from build123d import *

# Parameters (mm, degrees)
SKETCH1_R             = 41
BOSS_EXTRUDE1_DEPTH   = 34
SKETCH2_R             = 35
CUT_EXTRUDE1_DEPTH    = 21
CUT_EXTRUDE2_DEPTH    = 21
SKETCH6_R             = 11
BOSS_EXTRUDE2_DEPTH   = 26
ESBO_O1_R             = 3.25
CORTE_EXTRUS_O1_DEPTH = 15
ESBO_O2_W             = 0.9
ESBO_O2_H             = 31
CORTE_EXTRUS_O4_DEPTH = 12.8


with BuildPart() as part:
    # Sketch1 → Boss-Extrude1 (new body)
    with BuildSketch(Plane(origin=(0, 0, 0), x_dir=(1, 0, 0), z_dir=(0, 1, 0))):
        with Locations(Location((0, 0, 0), (0, 0, 270))):
            Circle(SKETCH1_R)
    extrude(amount=BOSS_EXTRUDE1_DEPTH)

    # Sketch2 → Cut-Extrude1 (cut)
    with BuildSketch(Plane(origin=(0, 34, 0), x_dir=(1, 0, 0), z_dir=(0, 1, 0))):
        with Locations(Location((0, 0, 0), (0, 0, 270))):
            Circle(SKETCH2_R)
    extrude(amount=-CUT_EXTRUDE1_DEPTH, mode=Mode.SUBTRACT)

    # Sketch3 → Cut-Extrude2 (cut)
    with BuildSketch(Plane.XZ):
        with BuildLine():
            Line((-4.632760116, 31.662873112), (-4.875607394, 23.89373544))
            ThreePointArc((-4.875607394, 23.89373544), (-10.738660694, 14.77258834), (-21.225170188, 12.015082756))
            Line((-21.225170188, 12.015082756), (-28.681580191, 14.190382579))
            ThreePointArc((-28.681580191, 14.190382579), (-18.809128073, 25.88854382), (-4.632760116, 31.662873112))
        make_face()
        with BuildLine():
            Line((28.681580191, 14.190382579), (21.217647246, 12.020548493))
            ThreePointArc((21.217647246, 12.020548493), (10.731137752, 14.778054077), (4.868084452, 23.899201177))
            Line((4.868084452, 23.899201177), (4.632760116, 31.662873112))
            ThreePointArc((4.632760116, 31.662873112), (18.809128073, 25.88854382), (28.681580191, 14.190382579))
        make_face()
        with BuildLine():
            Line((22.358951525, -22.892734365), (17.988834553, -16.464627908))
            ThreePointArc((17.988834553, -16.464627908), (17.370868563, -5.639248633), (24.23381184, 2.755435876))
            Line((24.23381184, 2.755435876), (31.544783405, 5.378349186))
            ThreePointArc((31.544783405, 5.378349186), (30.433808521, -9.88854382), (22.358951525, -22.892734365))
        make_face()
        with BuildLine():
            Line((-14.862988196, -28.338870512), (-10.099936075, -22.196248152))
            ThreePointArc((-10.099936075, -22.196248152), (0.004649434, -18.263301403), (10.109234942, -22.196248152))
            Line((10.109234942, -22.196248152), (14.862988196, -28.338870512))
            ThreePointArc((14.862988196, -28.338870512), (0, -32), (-14.862988196, -28.338870512))
        make_face()
        with BuildLine():
            Line((-31.544783405, 5.378349186), (-24.230938331, 2.746592128))
            ThreePointArc((-24.230938331, 2.746592128), (-17.367995055, -5.648092381), (-17.985961045, -16.473471657))
            Line((-17.985961045, -16.473471657), (-22.358951525, -22.892734365))
            ThreePointArc((-22.358951525, -22.892734365), (-30.433808521, -9.88854382), (-31.544783405, 5.378349186))
        make_face()
    extrude(amount=-CUT_EXTRUDE2_DEPTH, mode=Mode.SUBTRACT)

    # Sketch5 → Cut-Revolve1 (revolve, cut)
    with BuildSketch(Plane.XY, mode=Mode.PRIVATE) as cut_revolve1_sk:
        with BuildLine():
            Line((28, 0), (32, 0))
            Line((32, 0), (32, 4))
            ThreePointArc((32, 4), (30.828427125, 1.171572875), (28, 0))
        make_face()
        Polygon((0, 0), (0, 2.5), (9, 2.5), (9, 4), (12.5, 4), (14, 0), align=None)
    revolve(cut_revolve1_sk.sketch.rotate(Axis((0, 34, 0), (0, -1, 0)), 90), axis=Axis((0, 34, 0), (0, -1, 0)), mode=Mode.SUBTRACT)

    # Sketch6 → Boss-Extrude2 (add)
    with BuildSketch(Plane(origin=(0, 13, 0), x_dir=(1, 0, 0), z_dir=(0, 1, 0))):
        with Locations(Location((0, 0, 0), (0, 0, 90))):
            Circle(SKETCH6_R)
    extrude(amount=BOSS_EXTRUDE2_DEPTH)

    # Esboço1 → Corte-extrusão1 (cut)
    with BuildSketch(Plane(origin=(0, 39, 0), x_dir=(1, 0, 0), z_dir=(0, 1, 0))):
        with Locations(Location((0, 0, 0), (0, 0, 270))):
            Circle(ESBO_O1_R)
    extrude(amount=-CORTE_EXTRUS_O1_DEPTH, mode=Mode.SUBTRACT)

    # Esboço2 → Corte-Revolução1 (revolve, cut)
    with BuildSketch(Plane.XY, mode=Mode.PRIVATE) as corte_revolu_o1_sk:
        with Locations((-40.55, 17)):
            Rectangle(ESBO_O2_W, ESBO_O2_H)
    revolve(corte_revolu_o1_sk.sketch.rotate(Axis((0, -9.512295102, 0), (0, 1, 0)), 270), axis=Axis((0, -9.512295102, 0), (0, 1, 0)), mode=Mode.SUBTRACT)

    # Esboço3 → Corte-extrusão4 (cut)
    with BuildSketch(Plane(origin=(0, 39, 0), x_dir=(1, 0, 0), z_dir=(0, 1, 0))):
        with BuildLine():
            Line((-1.925, 2.618563538), (-1.925, 3.449184686))
            ThreePointArc((-1.925, 3.449184686), (0, 3.95), (1.925, 3.449184686))
            Line((1.925, 3.449184686), (1.925, 2.618563538))
            ThreePointArc((1.925, 2.618563538), (0, 3.25), (-1.925, 2.618563538))
        make_face()
    extrude(amount=-CORTE_EXTRUS_O4_DEPTH, mode=Mode.SUBTRACT)


solid = part.part
Geometry: final body of the model. Coordinates: model frame, mm. A direction names the side the tool comes from. Coordinates: 2 decimals unless noted, no trailing zeros. Order: outer loops, then holes, each group sorted by start corner. A loop starts at its lowest first (then second) coordinate and runs counter-clockwise, first axis right, second up. Notation, with made-up numbers: M 1,-17 L 52,-17 A15 cw 52,4 Z; hole C 16.5,46 d2. An arc over 180 degrees is marked long. One line per question, with ' | ' between items. Start each with the question number.
Item 1: Cut plane B-B, the plane z = -36. Return the cut outline in (x, y), then the cut area to 3 significant figures.
Item 2: Set-up query: faces 1 (the flat face through (-3, 4, 9)), 2 (the flat face through (20.2, 6.41, -19.72)), 3 (the flat face through (39.3, 32.5, -8.9)), 4 (the cylindrical face through (-21, 24, -28)). Return all of +Z, -Z, +X, -X, +Y, -Y with unobstructed straight access to the full face (end or side cutting, diameter ignored); none if empty.
Item 3: Cut plane A-A, the plane z = -15. Return the cut outline in (x, y), then the cut area to 3 significant figures.
Item 4: Cut plane D-D, the plane z = 20.5. Return the cut outline in (x, y), then the cut area to 3 significant figures.
Item 5: Pin query (flat end, axial travel): pin 1 Ø1.5 at (y, z) = (31, 26.5) entering from +X; pin 2 Ø6 at (x, y) = (8.5, 13) entering from +Z; pin 3 Ø1.5 at (x, z) = (0, -3) entering from +Y. Return the tip coordinate at first contact, or that it passes through.
Item 6: Cut plane C-C, the plane x = 6. Count the separate pieces of the cut face and the enclosed holes in it, then the cut area to 3 significant figures.
Item 7: Draft query along Z for faces 5 (the flat face through (0.1, 0, -14.4)), 6 (the cylindrical face through (-1.245, 31.605, 3.002)), 7 (the cylindrical face through (-40, 1, -9)). Return one class per face: released by +Z, released by -Z, zero draft, split by the parting line, or undercut.
Item 8: Ray query, probe 1 along X at (y, z) = (31.75, 0); probe 2 along X at (y, z) = (21, 0); probe 3 along X at (y, z) = (9, -17.5). Return the intervals inside material, ascending. Write a range as [from, to].
A:
1) outline: M -19.62,0 L 19.62,0 L 19.62,1.5 L 17.66,1.5 L 17.66,32.5 L 19.62,32.5 L 19.62,34 L -19.62,34 L -19.62,32.5 L -17.66,32.5 L -17.66,1.5 L -19.62,1.5 Z | area: 1,210 mm2
2) face 1: -Y | face 2: +Y, -Y | face 3: none | face 4: +Y
3) outline: M -38.16,0 L -28.27,0 L -28.27,13 L -31.62,13 L -31.62,34 L -38.16,34 L -38.16,32.5 L -37.19,32.5 L -37.19,1.5 L -38.16,1.5 Z; M -17.41,0 L 17.41,0 L 17.41,13 L -17.41,13 Z; M 28.27,0 L 38.16,0 L 38.16,1.5 L 37.19,1.5 L 37.19,32.5 L 38.16,32.5 L 38.16,34 L 31.62,34 L 31.62,13 L 28.27,13 Z | area: 924 mm2
4) outline: M -35.51,0 L -24.57,0 L -24.57,13 L -28.37,13 L -28.37,34 L -35.51,34 L -35.51,32.5 L -34.46,32.5 L -34.46,1.5 L -35.51,1.5 Z; M -6,0 L 6,0 L 6,13 L -6,13 Z; M 24.57,0 L 35.51,0 L 35.51,1.5 L 34.46,1.5 L 34.46,32.5 L 35.51,32.5 L 35.51,34 L 28.37,34 L 28.37,13 L 24.57,13 Z | area: 675 mm2
5) pin 1: stops at x = 30.74 | pin 2: stops at z = 39.72 | pin 3: stops at y = 26.2
6) separate pieces: 3 | enclosed holes: 0 | area: 1,360 mm2
7) face 5: zero draft | face 6: undercut | face 7: split by the parting line
8) probe 1: x = [-40.1, -35], [-11, -3.25], [3.25, 11], [35, 40.1] | probe 2: x = [-40.1, -35], [-11, 11], [35, 40.1] | probe 3: x = [-36.08, -26.79], [-18.69, 18.69], [26.79, 36.08]
